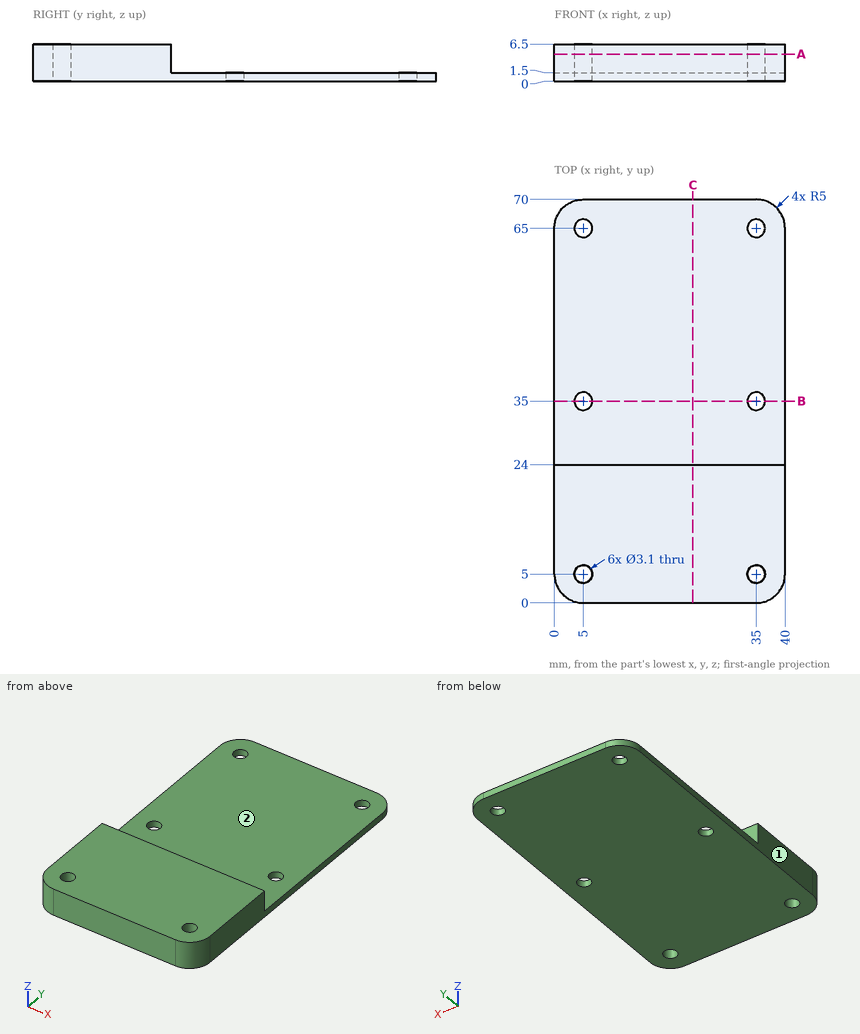
Geometry check sheet. Reference: drawing and pictorial views, mm from the part's lowest x, y, z. A direction names the side the tool comes from. Coordinates: 2 decimals unless noted, no trailing zeros. Loops run counter-clockwise (first coordinate to the right, second up) from the corner with the lowest first, then second, coordinate; pieces in that order, holes last.
1) Gauge pin test, flat ends, axial feed: pin 1 (3 mm diameter, centred on x = 5, y = 65, fed in from +Z); pin 2 (2.5 mm diameter, centred on x = 20.5, z = 4, fed in from +Y); pin 3 (20 mm diameter, centred on x = 13.5, y = 37.5, fed in from +Z). Record the tip position at first contact, or that the pin passes through.
2) Sectioned sample at C-C (x = 24). Record the boundary of the cut face in (y, z).
3) Access from +Z, -Z, +X, -X, +Y, -Y to the whole of each face (thin tool, end or side, straight path). Record for the marked faces 1 and 2.
4) Sectioned sample at A-A (z = 4.75). Record the boundary of the cut face in (x, y).
5) Material ranges on probe 1 along Y at (x, z) = (5, 0.45); probe 2 along X at (y, z) = (65, 0.3); probe 3 along Y at (x, z) = (6, 0.75), recorded low to high.
6) Sectioned sample at B-B (y = 35). Record the boundary of the cut face in (x, z).
Check sheet entries:
1. pin 1: passes through
1. pin 2: stops at y = 24
1. pin 3: stops at z = 1.5
2. outline: (0, 0) - (70, 0) - (70, 1.5) - (24, 1.5) - (24, 6.5) - (0, 6.5) - close
3. face 1: +Z, -Z, -X, +Y, -Y
3. face 2: +Z, +X, -X, +Y
4. outline: (0, 5) arc R5 ccw to (5, 0) - (35, 0) arc R5 ccw to (40, 5) - (40, 24) - (0, 24) - close; hole circle Ø3.1 at (5, 5); hole circle Ø3.1 at (35, 5)
5. probe 1: y = 0 to 3.45, 6.55 to 33.45, 36.55 to 63.45, 66.55 to 70
5. probe 2: x = 0 to 3.45, 6.55 to 33.45, 36.55 to 40
5. probe 3: y = 0 to 3.82, 6.18 to 33.82, 36.18 to 63.82, 66.18 to 70
6. outline: (0, 0) - (3.45, 0) - (3.45, 1.5) - (0, 1.5) - close; (6.55, 0) - (33.45, 0) - (33.45, 1.5) - (6.55, 1.5) - close; (36.55, 0) - (40, 0) - (40, 1.5) - (36.55, 1.5) - close
